```python
from build123d import *

# Parameters (mm, degrees)
F2_DEPTH = 101.6


# Not quite as in the source:
# - a variable given as a bare number and used for a length is read in inches; the dataset says mm whatever the document's units were


with BuildPart() as f2:
    # F1 (on Right) → F2 (new body, symmetric)
    with BuildSketch(Plane.YZ):
        with BuildLine():
            Line((44.45, 63.5), (-44.45, 63.5))
            ThreePointArc((-44.45, 63.5), (-57.9203841816, 57.9203841816), (-63.5, 44.45))
            Line((-63.5, 44.45), (-63.5, -44.45))
            ThreePointArc((-63.5, -44.45), (-57.9203841816, -57.9203841816), (-44.45, -63.5))
            Line((-44.45, -63.5), (44.45, -63.5))
            ThreePointArc((44.45, -63.5), (57.9203841816, -57.9203841816), (63.5, -44.45))
            Line((63.5, -44.45), (63.5, 44.45))
            ThreePointArc((63.5, 44.45), (57.9203841816, 57.9203841816), (44.45, 63.5))
        make_face()
        with BuildLine():
            ThreePointArc((-53.975, 44.45), (-51.1851920908, 51.1851920908), (-44.45, 53.975))
            Line((-44.45, 53.975), (44.45, 53.975))
            ThreePointArc((44.45, 53.975), (51.1851920908, 51.1851920908), (53.975, 44.45))
            Line((53.975, 44.45), (53.975, -44.45))
            ThreePointArc((53.975, -44.45), (51.1851920908, -51.1851920908), (44.45, -53.975))
            Line((44.45, -53.975), (-44.45, -53.975))
            ThreePointArc((-44.45, -53.975), (-51.1851920908, -51.1851920908), (-53.975, -44.45))
            Line((-53.975, -44.45), (-53.975, 44.45))
        make_face(mode=Mode.SUBTRACT)
    extrude(amount=F2_DEPTH, both=True)


solid = f2.part
```
Verification items for the finished model (mm, model axes). A direction names the side the tool comes from. Coordinates: 2 decimals unless noted, no trailing zeros. Loops run counter-clockwise (first coordinate to the right, second up) from the corner with the lowest first, then second, coordinate; pieces in that order, holes last. Notation, with made-up numbers: (-38, -38.5) -> (-30, -38.5) arc R3 ccw to (-30, -33.5) -> close; hole circle Ø2 at (-27, 73.25). An arc over 180 degrees is marked (long way). Answer in a Markdown table with one row per item.
1) Scan lines: line 1 along Z through (x, y) = (79, 12.5) (3 decimals); line 2 along Z through (x, y) = (-72, -52). Record each from-to range of solid material in increasing order. Write a range as from..to.
The answers:
| item | result |
|---|---|
| line 1 | z = -63.5..-53.975, 53.975..63.5 |
| line 2 | z = -61.94..-50.26, 50.26..61.94 |
2) Access from +Z, -Z, +X, -X, +Y, -Y to the whole of each face (thin tool, end or side, straight path). Record for faces 5 (the face through (1, 1, -53.975)), 6 (the face through (1, -1, -63.5)).
The answers:
| item | result |
|---|---|
| face 5 | +X, -X |
| face 6 | -Z, +X, -X, +Y, -Y |
3) Draft check along Z on faces 1 (the face through (1, 53.975, 1)), 2 (the face through (1, -63.5, 1)), 3 (the face through (1.42, 57.77, -58.07)), 4 (the face through (1, 1, 63.5)). Enter one of: released by +Z, released by -Z, zero draft, split by the parting line, or undercut.
The answers:
| item | result |
|---|---|
| face 1 | undercut |
| face 2 | zero draft |
| face 3 | released by -Z |
| face 4 | released by +Z |
4) Section check C-C (x = 57). Record the cut outline in (y, z) (3 decimals), and give its area (3 significant figures).
The answers:
| item | result |
|---|---|
| outline | (-63.5, -44.45) arc R19.05 ccw to (-44.45, -63.5) -> (44.45, -63.5) arc R19.05 ccw to (63.5, -44.45) -> (63.5, 44.45) arc R19.05 ccw to (44.45, 63.5) -> (-44.45, 63.5) arc R19.05 ccw to (-63.5, 44.45) -> close; hole (-53.975, -44.45) arc R9.525 ccw to (-44.45, -53.975) -> (44.45, -53.975) arc R9.525 ccw to (53.975, -44.45) -> (53.975, 44.45) arc R9.525 ccw to (44.45, 53.975) -> (-44.45, 53.975) arc R9.525 ccw to (-53.975, 44.45) -> close |
| area | 4,240 mm2 |
5) Section check A-A (z = 10). Record the cut outline in (x, y) (3 decimals), and give its area (3 significant figures).
The answers:
| item | result |
|---|---|
| outline | (-101.6, -63.5) -> (101.6, -63.5) -> (101.6, -53.975) -> (-101.6, -53.975) -> close; (-101.6, 53.975) -> (101.6, 53.975) -> (101.6, 63.5) -> (-101.6, 63.5) -> close |
| area | 3,870 mm2 |
